from build123d import *

# Parameters (mm, degrees)
SKETCH1_R           = 19.25
SKETCH1_R_2         = 4
BOSS_EXTRUDE1_DEPTH = 4
SKETCH1_4_R         = 4
BOSS_EXTRUDE2_DEPTH = 19


with BuildPart() as part:
    # Sketch1 → Boss-Extrude1 (new body)
    with BuildSketch(Plane(origin=(0, 0, 0), x_dir=(1, 0, 0), z_dir=(0, 1, 0))):
        Circle(SKETCH1_R)
        with BuildLine():
            ThreePointArc((2, -16.5), (0, -18.5), (-2, -16.5))
            Line((-2, -16.5), (-2, -16.378339354))
            ThreePointArc((-2, -16.378339354), (-14.289419162, -8.25), (-15.184057953, 6.45711887))
            Line((-15.184057953, 6.45711887), (-15.289419162, 6.517949192))
            ThreePointArc((-15.289419162, 6.517949192), (-16.02146997, 9.25), (-13.289419162, 9.982050808))
            Line((-13.289419162, 9.982050808), (-13.184057953, 9.921220485))
            ThreePointArc((-13.184057953, 9.921220485), (0, 16.5), (13.184057953, 9.921220485))
            Line((13.184057953, 9.921220485), (13.289419162, 9.982050808))
            ThreePointArc((13.289419162, 9.982050808), (16.02146997, 9.25), (15.289419162, 6.517949192))
            Line((15.289419162, 6.517949192), (15.184057953, 6.45711887))
            ThreePointArc((15.184057953, 6.45711887), (16.167667677, 3.294923655), (16.5, 0))
            ThreePointArc((16.5, 0), (12.354149101, -10.937321427), (2, -16.378339354))
            Line((2, -16.378339354), (2, -16.5))
        make_face(mode=Mode.SUBTRACT)
        with BuildLine():
            ThreePointArc((-15.184057953, 6.45711887), (-14.289419162, -8.25), (-2, -16.378339354))
            Line((-2, -16.378339354), (-2, -13.96))
            ThreePointArc((-2, -13.96), (0, -11.96), (2, -13.96))
            Line((2, -13.96), (2, -16.378339354))
            ThreePointArc((2, -16.378339354), (12.354149101, -10.937321427), (16.5, 0))
            ThreePointArc((16.5, 0), (16.167667677, 3.294923655), (15.184057953, 6.45711887))
            Line((15.184057953, 6.45711887), (13.089714637, 5.247949192))
            ThreePointArc((13.089714637, 5.247949192), (10.357663829, 5.98), (11.089714637, 8.712050808))
            Line((11.089714637, 8.712050808), (13.184057953, 9.921220485))
            ThreePointArc((13.184057953, 9.921220485), (0, 16.5), (-13.184057953, 9.921220485))
            Line((-13.184057953, 9.921220485), (-11.094979939, 8.715090731))
            Line((-11.094979939, 8.715090731), (-11.089714637, 8.712050808))
            ThreePointArc((-11.089714637, 8.712050808), (-10.357663829, 5.98), (-13.089714637, 5.247949192))
            Line((-13.089714637, 5.247949192), (-15.184057953, 6.45711887))
        make_face()
        Circle(SKETCH1_R_2, mode=Mode.SUBTRACT)
    extrude(amount=-BOSS_EXTRUDE1_DEPTH)

    # Sketch1_4 → Boss-Extrude2 (add)
    with BuildSketch(Plane(origin=(0, 0, 0), x_dir=(1, 0, 0), z_dir=(0, 1, 0))):
        Circle(SKETCH1_4_R)
    extrude(amount=-BOSS_EXTRUDE2_DEPTH)

    # Sketch2 → Cut-Revolve4 (revolve, cut)
    with BuildSketch(Plane(origin=(0, 0, 0), x_dir=(0, 0, -1), z_dir=(1, 0, 0))):
        Polygon((0, -19), (0.8, -19), (0.8, -17), (1, 0), (0, 0), align=None)
    revolve(axis=Axis((0, 0, 0), (0, -1, 0)), mode=Mode.SUBTRACT)

    # Sketch5 → Cut-Revolve8 (revolve, cut)
    with BuildSketch(Plane.XY):
        Polygon((0, -7), (-2.55, -5.527756814), (-2.55, 0), (0, 0), align=None)
    revolve(axis=Axis((0, 0, 0), (0, -1, 0)), mode=Mode.SUBTRACT)


solid = part.part
Geometry: final body of the model. Coordinates: model frame, mm. A direction names the side the tool comes from. Coordinates: 2 decimals unless noted, no trailing zeros. Order: outer loops, then holes, each group sorted by start corner. A loop starts at its lowest first (then second) coordinate and runs counter-clockwise, first axis right, second up.
1) Draft query along Z for faces 1 (the cylindrical face through (-16.043, -1.972, -9.212)), 2 (the flat face through (1, -19, 0)), 3 (the cylindrical face through (-0.867, -11.395, 3.905)), 4 (the cylindrical face through (-1.18, -2.73, 2.26)). Return one class per face: released by +Z, released by -Z, zero draft, split by the parting line, or undercut.
Result sheet:
face 1: undercut
face 2: zero draft
face 3: split by the parting line
face 4: undercut
2) Ray query, probe 1 along Z at (x, y) = (0, -2.5); probe 2 along Z at (x, y) = (0, -4.2); probe 3 along Y at (x, z) = (16, 1.5). Return the intervals inside material, ascending.
Result sheet:
probe 1: z = -19.25 to -2.55, 2.55 to 11.96, 18.5 to 19.25
probe 2: z = -4 to -2.55, 2.55 to 4
probe 3: y = -4 to 0
3) Section C-C (x = 0). Give the number of separate pieces and of enclosed holes in the cut face, then the cut area to 3 significant figures.
Result sheet:
separate pieces: 3
enclosed holes: 0
area: 195 mm2
4) Section B-B (z = -8.25). Return loops of the section in (x, y), then the cut area to 3 significant figures.
Result sheet:
outline: (-17.39, -4) - (-16.29, -4) - (-16.29, 0) - (-17.39, 0) - close; (-10.54, -4) - (10.54, -4) - (10.54, 0) - (-10.54, 0) - close; (16.29, -4) - (17.39, -4) - (17.39, 0) - (16.29, 0) - close
area: 93.2 mm2
5) First-contact query: P1, Ø3, axis at x = -2.5, z = 13, coming from the +Y side; P2, Ø1.3, axis at y = -3, z = 15, coming from the +X side; P3, Ø1, axis at x = 0, z = 0, coming from the -Y side; P4, Ø4, axis at x = -10.5, y = -2.5, coming from the -Z side. Flat tips, straight axial feed; report the tip coordinate or a pass-through.
Result sheet:
P1: stops at y = 0
P2: stops at x = 12.83
P3: passes through
P4: stops at z = -17.27
6) Set-up query: faces 5 (the conical face through (-0.84, -11.66, 0.19)), 6 (the flat face through (-2, -2, 15)), 7 (the flat face through (4, 0, 0)). Return all of +Z, -Z, +X, -X, +Y, -Y with unobstructed straight access to the full face (end or side cutting, diameter ignored); none if empty.
Result sheet:
face 5: +Y
face 6: +Y, -Y
face 7: +Z, -Z, +X, -X, +Y
7) Section D-D (y = -8.75). Return loops of the section in (x, z), then the cut area to 3 significant figures.
Result sheet:
outline: circle Ø8 at (0, 0); hole circle Ø1.79 at (0, 0)
area: 47.7 mm2
8) Section A-A (y = -2.5). Return loops of the section in (x, z).
Result sheet:
outline: circle Ø38.5 at (0, 0); hole (-15.29, -6.52) arc R2 ccw to (-13.29, -9.98) - (-11.09, -8.71) arc R2 ccw to (-13.09, -5.25) - close; hole circle Ø5.1 at (0, 0); hole (-2, 13.96) arc R2 ccw to (2, 13.96) - (2, 16.5) arc R2 ccw to (-2, 16.5) - close; hole (11.09, -8.71) - (13.29, -9.98) arc R2 ccw to (15.29, -6.52) - (13.09, -5.25) arc R2 ccw to start
